Work out the finished part from the listing and answer in its coordinate system (mm). Face numbers are marked on the shaded views. A direction names the side the tool comes from. Round coordinates to 2 decimals unless told otherwise and drop trailing zeros. Order: outer loops, then holes, each group sorted by start corner. A loop starts at its lowest first (then second) coordinate and runs counter-clockwise, first axis right, second up. Notation, with made-up numbers: (12.5, 34) - (51.5, 34) arc R21 cw to (51.5, 72) - close; hole circle Ø10 at (25.5, -13.75). An arc over 180 degrees is marked (long way). Answer in a Markdown table with one row per item.
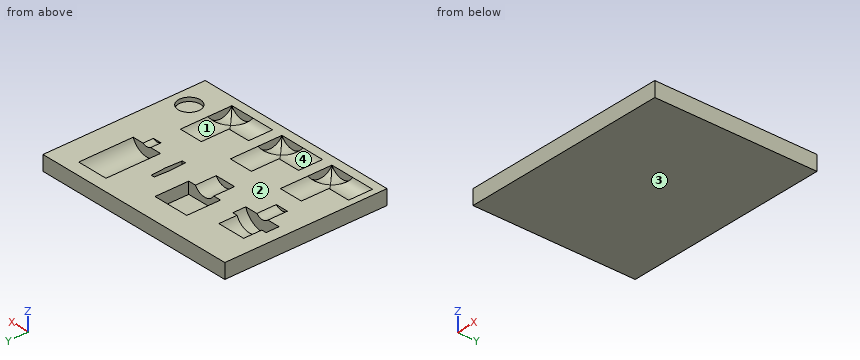
from build123d import *

# Parameters (mm, degrees)
F0_W      = 160
F0_H      = 125
F1_DEPTH  = 16.5
F2_W      = 37
F2_H      = 10.5
F4_W      = 10.5
F4_H      = 41
F6_W      = 10.5
F6_H      = 41
F8_W      = 10.5
F8_H      = 41
F10_R     = 8.5
F11_DEPTH = 8
F14_W     = 9.5
F14_H     = 16
F17_DEPTH = 14
F20_W     = 160
F20_H     = 5
F21_DEPTH = 150
F24_W     = 18.4661853126
F24_H     = 1.2669073437
F24_W_2   = 1.2669073437
F24_H_2   = 18.4661853126
F25_DEPTH = 10
F27_START = -10.5
F27_DEPTH = 1


with BuildPart() as f1:
    # F0 (on Top) → F1 (new body)
    with BuildSketch(Plane.XY):
        with Locations((80, 62.5)):
            Rectangle(F0_W, F0_H)
    extrude(amount=-F1_DEPTH)

    # F2 (on face) → F3 (revolve, cut)
    with BuildSketch(Plane.XY):
        with Locations((23.5, 10.75)):
            Rectangle(F2_W, F2_H)
        with Locations((67.5, 10.75)):
            Rectangle(F2_W, F2_H)
        with Locations((111.5, 10.75)):
            Rectangle(F2_W, F2_H)
    revolve(axis=Axis((23.5, 16, 0), (1, 0, 0)), mode=Mode.SUBTRACT)

    # F4 (on face) → F5 (revolve, cut)
    with BuildSketch(Plane.XY):
        with Locations((36.75, 26)):
            Rectangle(F4_W, F4_H)
    revolve(axis=Axis((31.5, 26, 0), (0, 1, 0)), mode=Mode.SUBTRACT)

    # F6 (on face) → F7 (revolve, cut)
    with BuildSketch(Plane.XY):
        with Locations((80.75, 26)):
            Rectangle(F6_W, F6_H)
    revolve(axis=Axis((75.5, 26, 0), (0, 1, 0)), mode=Mode.SUBTRACT)

    # F8 (on face) → F9 (revolve, cut)
    with BuildSketch(Plane.XY):
        with Locations((124.75, 26)):
            Rectangle(F8_W, F8_H)
    revolve(axis=Axis((119.5, 26, 0), (0, 1, 0)), mode=Mode.SUBTRACT)

    # F10 (on face) → F11 (cut)
    with BuildSketch(Plane.XY):
        with Locations((145.7579010625, 24.7283919918)):
            Circle(F10_R)
    extrude(amount=-F11_DEPTH, mode=Mode.SUBTRACT)

    # F12 (on face) → F13 (revolve, cut)
    with BuildSketch(Plane.XY):
        Polygon((24, 75), (24, 60), (31, 60), (31, 75), (39.5, 75), (39.5, 85), (36, 85), (36, 99), (28.5, 99), (28.5, 113), (24, 113), (24, 99), (24, 85), align=None)
    revolve(axis=Axis((24, 92, 0), (0, 1, 0)), mode=Mode.SUBTRACT)

    # F14 (on face) → F15 (revolve, cut)
    with BuildSketch(Plane.XY):
        with Locations((72.75, 73)):
            Rectangle(F14_W, F14_H)
    revolve(axis=Axis((68, 73, 0), (0, 1, 0)), mode=Mode.SUBTRACT)

    # F16 (on face) → F17 (cut)
    with BuildSketch(Plane.XY):
        Polygon((54, 107), (54, 81), (58.5, 81), (77.5, 81), (82, 81), (82, 107), align=None)
    extrude(amount=-F17_DEPTH, mode=Mode.SUBTRACT)

    # F18 (on face) → F19 (revolve, cut)
    with BuildSketch(Plane.XY):
        Polygon((128, 73), (128, 65), (134, 65), (134, 73), (141, 73), (141, 115), (128, 115), align=None)
    revolve(axis=Axis((128, 94, 0), (0, 1, 0)), mode=Mode.SUBTRACT)

    # F20 (on Front) → F21 (cut)
    with BuildSketch(Plane.XZ):
        with Locations((80, -2.5)):
            Rectangle(F20_W, F20_H)
    extrude(amount=-F21_DEPTH, mode=Mode.SUBTRACT)

    # F22 (on face) → F23 (revolve, cut)
    with BuildSketch(Plane.XY.offset(-5)):
        Polygon((98.6288933514, 93), (98, 81), (102, 81), (101.3711066486, 93), align=None)
    revolve(axis=Axis((100, 81, -5), (1, 0, 0)), mode=Mode.SUBTRACT)

    # F24 (on face) → F25 (join)
    with BuildSketch(Plane.XY.offset(-5)):
        with Locations((31.5, 6.1334536718)):
            Rectangle(F24_W, F24_H)
        with Locations((41.3665463282, 16)):
            Rectangle(F24_W_2, F24_H_2)
        with Locations((85.3665463282, 16)):
            Rectangle(F24_W_2, F24_H_2)
        with Locations((75.5, 6.1334536718)):
            Rectangle(F24_W, F24_H)
        with Locations((129.3665463282, 16)):
            Rectangle(F24_W_2, F24_H_2)
        with Locations((119.5, 6.1334536718)):
            Rectangle(F24_W, F24_H)
    extrude(amount=-F25_DEPTH)

    # F26 (on face) → F27 (join)
    with BuildSketch(Plane.XY.offset(-5).offset(F27_START)):
        Polygon((101.528329799, 90.0000035763), (98.471670201, 90.0000035763), (98, 81), (98.3558213304, 74.210524559), (101.6441786696, 74.210524559), (102, 81), align=None)
    extrude(amount=-F27_DEPTH)


solid = f1.part
1) Find section A-A, the plane x = 80. Give the vertices of the cut face in (y, z), then the cut area to 3 significant figures.
Filled in:
| item | result |
|---|---|
| outline | (0, -16.5) - (125, -16.5) - (125, -5) - (107, -5) - (107, -14) - (81, -14) - (81, -5) - (46.5, -5) - (46.5, -9.49) - (20.5, -9.49) arc R10.5 cw to (11.5, -9.49) - (6.77, -9.49) - (6.77, -5) - (0, -5) - close |
| area | 1,020 mm^2 |
2) Find the intervals of material crossed by probe 1 along Y at (x, z) = (77, -8); probe 2 along Y at (x, z) = (35, -6.25); probe 3 along X at (y, z) = (26, -6), in increasing order. Write a range as from..to.
Filled in:
| item | result |
|---|---|
| probe 1 | y = 0..6.77, 46.5..81, 107..125 |
| probe 2 | y = 0..6.77, 46.5..75, 85..125 |
| probe 3 | x = 0..22.88, 40.12..66.88, 84.12..110.88, 128.12..137.35, 154.16..160 |
3) The mould has two halves that part along Y. Classify the marked faces 3 and 4: released by +Y, released by -Y, zero draft, split by the parting line, or undercut.
Filled in:
| item | result |
|---|---|
| face 3 | zero draft |
| face 4 | undercut |
4) This flat-tipped pin is pushed along its axis until it touches: pin 1 (13 mm diameter, centred on x = 69.5, y = 96.5, fed in from +Z). Where does it stop, or does it pass through?
Filled in:
| item | result |
|---|---|
| pin 1 | stops at z = -14 |
5) Which of the six approach directions +Z, -Z, +X, -X, +Y, -Y give full straight-line access (tool end or side, diameter ignored) to the marked faces 1 and 2?
Filled in:
| item | result |
|---|---|
| face 1 | +Z |
| face 2 | +Z, +X, -X, +Y, -Y |
